Build history of the part. All positions in model axes, mm. A direction names the side the tool comes from. Round coordinates to 2 decimals unless told otherwise and drop trailing zeros. Loops run counter-clockwise (first coordinate to the right, second up) from the corner with the lowest first, then second, coordinate; pieces in that order, holes last. Notation, with made-up numbers: (0.25, 13) - (21.25, 13) arc R9 ccw to (21.25, 23) - close; hole circle Ø11 at (69, 19). An arc over 180 degrees is marked (long way). Use a Markdown table: item, result.
Autodesk Inventor part; units mm, degrees
ref_plane "YZ Plane" through (0, 0, 0) normal (1, 0, 0) x (0, 1, 0)
ref_plane "XZ Plane" through (0, 0, 0) normal (0, 1, 0) x (-1, 0, 0)
ref_plane "XY Plane" through (0, 0, 0) normal (0, 0, 1) x (1, 0, 0)
sketch "Sketch1" plane through (0, 0, 0) normal (1, 0, 0) x (0, 1, 0)
  line L0 (0, 0) -> (0, -104)
  line L1 (79.3684, 0) -> (0, -104)
  line L2 (79.3684, 0) -> (0, 0)
  line L3 (0, -104) -> (0, -104)
  line L4 (0, -104) -> (0, -106)
  line L5 (0, -106) -> (0, -106)
  line L6 (12, -88.2759) -> (12, -121.4374)
  line L7 (17, -106) -> (0, -106)
  line L8 (17, -104) -> (0, -104)
  line L9 (85.6581, 0) -> (17, -89.9658)
  line L10 (105.5294, 0) -> (79.3684, 0)
  line L11 (17, -89.9658) -> (17, -119.3457)
  circle A0 centre (12, -106) radius 2
  point P0 (12, -104)
  point P1 (14, -106)
  dimension "d5" = 79.3684
  dimension "d6" = 104
  dimension "d7" = 12
  dimension "d8" = 88.2759
  dimension "d9" = 0
  dimension "d11" = 2
  dimension "d12" = 5
  dimension "d13" = 5
extrude "Extrusion1" add sketch "Sketch1" along normal blind 2 contours L10 L9 L11 L8 L6 L1 | L8 L11 L7 A0
sketch "Sketch2" plane through (2, 0, 0) normal (1, 0, 0) x (0, 0, -1)
  line L0 (0, 85.6581) -> (0, 79.3684)
  line L1 (0, 80.6581) -> (89.9658, 12)
  line L2 (88.2759, 12) -> (104, 12)
  line L3 (0, 79.3684) -> (88.2759, 12)
  line L4 (102.4983, 12) -> (102.4983, 15.9748)
  line L5 (89.9658, 17) -> (0, 85.6581)
  line L6 (106, 14) -> (106, 17)
  line L7 (106, 15.9748) -> (91.3092, 15.9748)
  line L8 (0, 85.6581) -> (91.3092, 15.9748)
  line L9 (106, 15.9748) -> (106, 17)
  line L10 (106, 17) -> (89.9658, 17)
  line L11 (106, 15.9748) -> (106, 17)
  line L12 (106, 17) -> (89.9658, 17)
  point P0 (0, 0)
  dimension "d18" = 5
  dimension "d19" = 3.9748
  dimension "d20" = 3.9748
extrude "Extrusion2" cut sketch "Sketch2" against normal blind 2 contours L1 L2 L3 L0 | L10 L6 L7 L8
sketch "Sketch3" plane through (2, 0, 0) normal (1, 0, 0) x (0, 0, -1)
  line L0 (91.3092, 15.9748) -> (0, 85.6581)
  line L1 (0, 85.6581) -> (91.3092, 15.9748)
  line L2 (91.3092, 15.9748) -> (106, 15.9748)
  line L3 (91.3092, 15.9748) -> (106, 15.9748)
  arc A0 (106, 14) -> (104, 12) centre (106, 12) ccw
  line L4 (106, 15.9748) -> (106, 14)
  circle A1 centre (106, 12) radius 2
  line L5 (89.9658, 12) -> (104, 12)
  line L6 (89.9658, 12) -> (104, 12)
  line L7 (0, 85.6581) -> (0, 80.6581)
  line L8 (0, 85.6581) -> (0, 80.6581)
  line L9 (0, 80.6581) -> (89.9658, 12)
  line L10 (0, 83.1581) -> (-58.5, 83.1581)
  line L11 (0, 85.6581) -> (0, 80.6581)
  line L12 (-58.5, 83.1581) -> (-58.5, 115.0333)
  line L13 (106, 14) -> (104, 14)
  line L14 (104, 14) -> (104, -16)
  line L15 (104, -16) -> (106, -16)
  line L16 (106, -16) -> (106, 14)
  point P0 (0, 0)
  dimension "d21" = 58.5
  dimension "d32" = 30
revolve "Revolution1" add sketch "Sketch3" angle 90 about axis through (2, 83.1581, 58.5) along (0, -1, 0) contours L2 L4 L13 L14 L5 L9 L7 L0 | L16 A1 A0 | A0 L14 L13 | A1 L16 L15 L14
sketch "Sketch14" plane through (166.5, -16, 58.5) normal (0, 0, 1) x (1, 0, 0)
  line L0 (-14.6908, 31.9748) -> (-106, 101.6581)
  line L1 (-106, 96.6581) -> (-16.0342, 28)
  line L2 (-106, 101.6581) -> (-106, 96.6581)
  line L3 (-16.0342, 28) -> (-2, 28)
  line L4 (-106, 96.6581) -> (-16.0342, 28)
  point P0 (-166.5, 16)
sketch "Sketch4" plane through (60.5, 80.6581, 58.5) normal (0, 0, 1) x (1, 0, 0)
  line L0 (0, 5) -> (0, 0)
  line L1 (0, 5) -> (0, 0)
  line L2 (0, 0) -> (89.9658, -68.6581)
  line L3 (0, 0) -> (89.9658, -68.6581)
  line L4 (89.9658, -68.6581) -> (104, -68.6581)
  line L5 (89.9658, -68.6581) -> (104, -68.6581)
  line L6 (106, -66.6581) -> (106, -64.6834)
  line L7 (106, -66.6581) -> (106, -64.6834)
  line L8 (91.3092, -64.6834) -> (0, 5)
  line L9 (106, -64.6834) -> (91.3092, -64.6834)
  line L10 (91.3092, -64.6834) -> (0, 5)
  arc A0 (106, -66.6581) -> (104, -68.6581) centre (106, -68.6581) ccw
  circle A1 centre (106, -68.6581) radius 2
  point P0 (-60.5, -80.6581)
extrude "Extrusion3" add sketch "Sketch4" along normal blind 2 contours L8 L9 L6 A0 L4 L2 L0
sketch "Sketch5" plane through (60.5, 80.6581, 60.5) normal (0, 0, 1) x (1, 0, 0)
  line L0 (0, 5) -> (0, 0)
  line L1 (0, 2.5) -> (90.621, -66.6581)
  line L2 (-58.5, -66.6581) -> (106, -66.6581)
  line L3 (91.3092, -64.6834) -> (0, 5)
  line L4 (90.621, -66.6581) -> (106, -66.6581)
  line L5 (106, -66.6581) -> (106, -64.6834)
  line L6 (106, -64.6834) -> (91.3092, -64.6834)
  line L7 (106, -64.6834) -> (91.3092, -64.6834)
  line L8 (-58.5, 5) -> (0, 5)
  line L9 (91.3092, -64.6834) -> (0, 5)
  line L10 (0, 5) -> (0, 2.5)
  point P0 (-60.5, -80.6581)
extrude "Extrusion4" cut sketch "Sketch5" against normal blind 2
sketch "Sketch6" plane through (0, 0, 0) normal (-1, 0, 0) x (0, 0, 1)
  line L0 (0, 85.6581) -> (0, 80.6581)
  line L1 (0, 83.1581) -> (-90.621, 14)
  line L2 (-106, 14) -> (58.5, 14)
  line L3 (-91.3092, 15.9748) -> (0, 85.6581)
  line L4 (-106, 14) -> (-106, 15.9748)
  line L5 (-90.621, 14) -> (-106, 14)
  line L6 (-106, 14) -> (-106, 15.9748)
  line L7 (-106, 15.9748) -> (-91.3092, 15.9748)
  line L8 (0, 85.6581) -> (0, 83.1581)
  point P0 (0, 0)
extrude "Extrusion5" cut sketch "Sketch6" against normal blind 2
equation "\"d19\" = d20"
properties part number "Cover_v1"
Q1. Cut at C-C, the plane y = 28. List the corners of the cut face in (x, z), plus the area to 3 significant figures.
Results found:
| item | result |
|---|---|
| outline | (0, -72.28) - (2, -72.28) - (2, -75.55) arc R134.05 ccw to (136.05, 58.5) - (132.78, 58.5) - (132.78, 60.5) - (129.5, 60.5) - (129.5, 58.5) arc R127.5 cw to (2, -69) - (0, -69) - close |
| area | 1,360 mm2 |
Q2. Cut at B-B, the plane x = 154. List the corners of the cut face in (y, z), plus the area to 3 significant figures.
Results found:
| item | result |
|---|---|
| outline | (-16, -4.4) - (15.97, -4.4) - (15.97, 58.5) - (14, 58.5) - (14, 60.5) - (12, 60.5) - (12, 1.03) - (-16, 1.03) - close |
| area | 406 mm2 |
Q3. Cut at A-A, the plane y = 64.5. List the corners of the cut face in (x, z), plus the area to 3 significant figures.
Results found:
| item | result |
|---|---|
| outline | (0, -24.45) - (2, -24.45) - (2, -27.72) arc R86.22 ccw to (88.22, 58.5) - (84.95, 58.5) - (84.95, 60.5) - (81.67, 60.5) - (81.67, 58.5) arc R79.67 cw to (2, -21.17) - (0, -21.17) - close |
| area | 867 mm2 |
Q4. Probe line 1 (Y direction, x = 34.5, z = -98.5); line 2 (Y direction, x = 36.5, z = -34); line 3 (Z direction, x = 81, y = 2). List the from-to ranges inside material, lowest first.
Results found:
| item | result |
|---|---|
| line 1 | y = 12 to 15.97 |
| line 2 | y = 49.96 to 54.96 |
| line 3 | z = -85.79 to -83.5 |
Q5. Which spindle directions (+Z, -Z, +X, -X, +Y, -Y) get a long thin tool onto all of the face, cutting with end or side? Do faces 1 (the face through (0.99, 49.06, -44.68)), 2 (the face through (113, 45, 58.5)), 3 (the face through (106, 12, -53)). Say none if no direction does.
Results found:
| item | result |
|---|---|
| face 1 | -Z, -X, +Y |
| face 2 | +Z, +X, +Y |
| face 3 | +Z, -X, -Y |
Q6. Cut at D-D, the plane y = -2.5. List the corners of the cut face in (x, z), plus the area to 3 significant figures.
Results found:
| item | result |
|---|---|
| outline | (2, -106) arc R164.5 ccw to (166.5, 58.5) - (164.5, 58.5) arc R162.5 cw to (2, -104) - close |
| area | 514 mm2 |
Q7. Drop flat-ended pins along their axis: pin 1 (10 mm diameter, centred on x = 42.5, z = -37.5, fed in from +Y); pin 2 (8 mm diameter, centred on x = 92, z = -22.5, fed in from +Y); pin 3 (2 mm diameter, centred on x = 165, y = 5, fed in from +Z); pin 4 (3 mm diameter, centred on x = 133, z = -46, fed in from -Y). Give the stop position or say it passes through.
Results found:
| item | result |
|---|---|
| pin 1 | stops at y = 54.6 |
| pin 2 | stops at y = 40.95 |
| pin 3 | stops at z = 58.5 |
| pin 4 | passes through |
